Geometry: final body of the model. Coordinates: model frame, mm. A direction names the side the tool comes from. Give positions to 0.01 mm unless a question says otherwise; leave off trailing zeros. Loops run counter-clockwise (first coordinate to the right, second up) from the corner with the lowest first, then second, coordinate; pieces in that order, holes last.
1. Section B-B, the plane x = -3.75. Output: boundary loops of the cut face in (y, z), then the cut area to 3 significant figures.
2. Section C-C, the plane y = 3.5. Output: boundary loops of the cut face in (x, z), then the cut area to 3 significant figures.
3. Section A-A, the plane z = -2.5. Output: boundary loops of the cut face in (x, y), then the cut area to 3 significant figures.
4. Material intervals for line 1 along X through (y, z) = (7.25, -5.5); line 2 along Z through (x, y) = (-2.5, 7); line 3 along Y through (x, z) = (-4.75, -4), sorted ascending.
5. Section D-D, the plane y = 7.75. Output: boundary loops of the cut face in (x, z).
6. Access query for faces 4 (the face through (-1, 8, -5)), 5 (the face through (-4.4, 4, -5)). Directions: +Z, -Z, +X, -X, +Y, -Y. A direction counts if a zero-diameter tool reaches every point of the face in a straight line with its end or side. Return the directions, or none.
7. Draft query along X for faces 1 (the face through (-3, 4, -2)), 2 (the face through (-1, 0, -5)), 3 (the face through (-6.4, 4, -4)). Return one class per face: +X half, -X half, draft (parallel to the pull), parting line (faces both ways), or undercut.
from build123d import *

# Parameters (mm, degrees)
BOSS_EXTRUDE1_DEPTH = 8
FILLET1_R           = 0.4


with BuildPart() as part:
    # Sketch1 → Boss-Extrude1 (new body)
    with BuildSketch(Plane(origin=(0, 0, 0), x_dir=(1, 0, 0), z_dir=(0, 1, 0))):
        Polygon((0, 0), (-6.4, 0), (-6.4, 9), (-4.4, 9), (-4.4, 2), (-2, 2), (-2, 9), (0, 9), align=None)
    extrude(amount=BOSS_EXTRUDE1_DEPTH)

    # Fillet1
    fillet1_edges = [part.edges().sort_by_distance(p)[0] for p in [
        (-3.2, 0, -2),
        (-2, 0, -5.5),
        (-1, 0, -9),
        (0, 0, -4.5),
        (-2, 8, -5.5),
        (0, 4, 0),
        (-6.4, 4, 0),
        (-6.4, 4, -9),
        (-4.4, 4, -9),
        (-2, 4, -9),
        (0, 4, -9),
        (-3.2, 8, -2),
        (-4.4, 8, -5.5),
        (-5.4, 8, -9),
        (-6.4, 8, -4.5),
        (-3.2, 8, 0),
        (0, 8, -4.5),
        (-3.2, 0, 0),
        (-1, 8, -9),
        (-6.4, 0, -4.5),
        (-5.4, 0, -9),
        (-4.4, 0, -5.5),
    ]]
    fillet(fillet1_edges, radius=FILLET1_R)


solid = part.part
Answers below:
1. outline: (0, -1.6) arc R0.4 ccw to (0.4, -2) - (7.6, -2) arc R0.4 ccw to (8, -1.6) - (8, -0.4) arc R0.4 ccw to (7.6, 0) - (0.4, 0) arc R0.4 ccw to (0, -0.4) - close
1. area: 15.9 mm2
2. outline: (-6.4, -8.6) arc R0.4 ccw to (-6, -9) - (-4.8, -9) arc R0.4 ccw to (-4.4, -8.6) - (-4.4, -2) - (-2, -2) - (-2, -8.6) arc R0.4 ccw to (-1.6, -9) - (-0.4, -9) arc R0.4 ccw to (0, -8.6) - (0, -0.4) arc R0.4 ccw to (-0.4, 0) - (-6, 0) arc R0.4 ccw to (-6.4, -0.4) - close
2. area: 40.6 mm2
3. outline: (-6.4, 0.4) arc R0.4 ccw to (-6, 0) - (-4.8, 0) arc R0.4 ccw to (-4.4, 0.4) - (-4.4, 7.6) arc R0.4 ccw to (-4.8, 8) - (-6, 8) arc R0.4 ccw to (-6.4, 7.6) - close; (-2, 0.4) arc R0.4 ccw to (-1.6, 0) - (-0.4, 0) arc R0.4 ccw to (0, 0.4) - (0, 7.6) arc R0.4 ccw to (-0.4, 8) - (-1.6, 8) arc R0.4 ccw to (-2, 7.6) - close
3. area: 31.7 mm2
4. line 1: x = -6.4 to -4.4, -2 to 0
4. line 2: z = -2 to 0
4. line 3: y = 0 to 8
5. outline: (-6.37, -8.6) arc R0.37 ccw to (-6, -8.97) - (-4.8, -8.97) arc R0.37 ccw to (-4.43, -8.6) - (-4.43, -1.97) - (-1.97, -1.97) - (-1.97, -8.6) arc R0.37 ccw to (-1.6, -8.97) - (-0.4, -8.97) arc R0.37 ccw to (-0.03, -8.6) - (-0.03, -0.4) arc R0.37 ccw to (-0.4, -0.03) - (-6, -0.03) arc R0.37 ccw to (-6.37, -0.4) - close
6. face 4: +Z, -Z, +X, -X, +Y
6. face 5: -Z, +Y, -Y
7. face 1: undercut
7. face 2: draft
7. face 3: -X half
